Build history of the part. All positions in model axes, mm. Give positions to 0.01 mm unless a question says otherwise; leave off trailing zeros. Loops run counter-clockwise (first coordinate to the right, second up) from the corner with the lowest first, then second, coordinate; pieces in that order, holes last. Notation, with made-up numbers: (54, 35.25) -> (63, 35.25) arc R23 ccw to (63, 52.25) -> close; hole circle Ø1 at (47.25, 72). An arc over 180 degrees is marked (long way). Answer as a JSON object with one key per item and string values. Group by question number.
Q1. Drop flat-ended pins along their axis: pin 1 (2 mm diameter, centred on x = 2.5, z = -2, fed in from +Y); pin 2 (1.5 mm diameter, centred on y = -1.5, z = 4, fed in from +X); pin 3 (1 mm diameter, centred on y = -1, z = -3, fed in from +X); pin 4 (1.5 mm diameter, centred on y = -2.5, z = 3, fed in from -X). Give the stop position or say it passes through.
Q2. Band-saw the part on A-A, the plane x = 0. Write the cut outline in (y, z), plus the area to 3 significant figures.
Q3. Band-saw the part on C-C, the plane y = -4.5. Write the cut outline in (x, z), plus the area to 3 significant figures.
Q4. Wall check: probe 1 along Z at (x, y) = (0, -4); probe 2 along Z at (x, y) = (0.5, -0.75); probe 3 along Z at (x, y) = (3, -6.5). Give the ranges that are in metal, low to high. Write a range as from..to.
Q5. Two-plate mould, pull along X, no slides. Class faces 1 (the cylindrical face through (-1.08, -3.45, -4.88)), 2 (the flat face through (-0.1, 0, -2.2)), 3 (the cylindrical face through (0, -4, -2)): pulls with the +X half, pulls with the -X half, needs draft (parallel to the pull), parting line crosses it, or undercut.
Q6. Band-saw the part on B-B, the plane z = 0. Write the cut outline in (x, y).
from build123d import *

# Parameters (mm, degrees)
F0_R     = 5
F1_DEPTH = 8
F3_D     = 4
F4_SIZE  = 1


with BuildPart() as f1:
    # F0 (on Front) → F1 (new body)
    with BuildSketch(Plane.XZ):
        Circle(F0_R)
    extrude(amount=F1_DEPTH)

    # F3 (through all)
    with Locations(Plane.XZ.offset(8)):
        with Locations((0, 0)):
            Hole(F3_D / 2)

    # F4
    f4_edges = [f1.edges().sort_by_distance(p)[0] for p in [
        (-5, -8, 0),
    ]]
    chamfer(f4_edges, length=F4_SIZE)


solid = f1.part
Worked answers:
{
 "1": {"pin 1": "y = 0", "pin 2": "x = 3.8", "pin 3": "x = 4.33", "pin 4": "x = -4.47"},
 "2": {"outline": "(-8, -4) -> (-7, -5) -> (0, -5) -> (0, -2) -> (-8, -2) -> close; (-8, 2) -> (0, 2) -> (0, 5) -> (-7, 5) -> (-8, 4) -> close", "area": "47.0 mm2"},
 "3": {"outline": "circle Ø10 at (0, 0); hole circle Ø4 at (0, 0)", "area": "66.0 mm2"},
 "4": {"probe 1": "-5..-2, 2..5", "probe 2": "-4.97..-1.94, 1.94..4.97", "probe 3": "-4..4"},
 "5": {"face 1": "parting line crosses it", "face 2": "needs draft", "face 3": "undercut"},
 "6": {"outline": "(-5, -7) -> (-4, -8) -> (-2, -8) -> (-2, 0) -> (-5, 0) -> close; (2, -8) -> (4, -8) -> (5, -7) -> (5, 0) -> (2, 0) -> close"}
}
